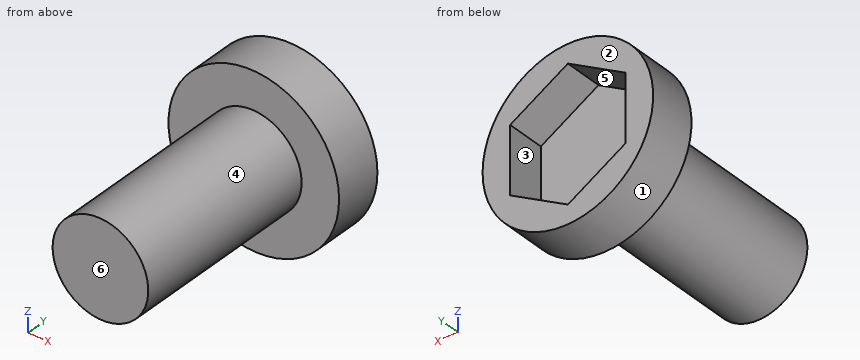
Autodesk Inventor part; units mm, degrees
ref_plane "YZ Plane" through (0, 0, 0) normal (1, 0, 0) x (0, 1, 0)
ref_plane "XZ Plane" through (0, 0, 0) normal (0, 1, 0) x (-1, 0, 0)
ref_plane "XY Plane" through (0, 0, 0) normal (0, 0, 1) x (1, 0, 0)
sketch "Sketch1" plane through (0, 0, 0) normal (0, 1, 0) x (-1, 0, 0)
  circle A0 centre (0, 0) radius 6.35
  dimension "d0" = 12.7
extrude "Extrusion1" add sketch "Sketch1" along normal blind 25.4
thread "Thread1"
sketch "Sketch2" plane through (0, 25.4, 0) normal (0, 1, 0) x (1, 0, 0)
  circle A0 centre (0, 0) radius 11.3208
extrude "Extrusion2" add sketch "Sketch2" along normal blind 6.35
sketch "Sketch3" plane through (0, 31.75, 0) normal (0, 1, 0) x (1, 0, 0)
  line L0 (0, 8.8433) -> (7.6585, 4.4216)
  line L1 (7.6585, 4.4216) -> (7.6585, -4.4216)
  line L2 (7.6585, -4.4216) -> (0, -8.8433)
  line L3 (0, -8.8433) -> (-7.6585, -4.4216)
  line L4 (-7.6585, -4.4216) -> (-7.6585, 4.4216)
  line L5 (-7.6585, 4.4216) -> (0, 8.8433)
  point P0 (0, 0)
  point P1 (0, 0)
extrude "Extrusion3" cut sketch "Sketch3" against normal blind 5.08
properties part number "bolttest"
Design review of the part built by this model. Coordinates are the model's own, in mm. Face numbers are marked on the shaded views. A direction names the side the tool comes from. Round coordinates to 2 decimals unless told otherwise and drop trailing zeros. Loops run counter-clockwise (first coordinate to the right, second up) from the corner with the lowest first, then second, coordinate; pieces in that order, holes last. Notation, with made-up numbers: (84.5, 47) -> (128.5, 47) arc R11 cw to (128.5, 55) -> close; hole circle Ø1 at (28, 72.25). An arc over 180 degrees is marked (long way). Use one line per item in the form item = value. Start each with the question number.
Q1. We need section B-B on z = 0. Give the boundary of the cut face in (x, y).
Q2. We need section C-C on y = 24. Give the boundary of the cut face in (x, z), then the cut area to 3 significant figures.
Q3. Machinability: for the marked faces 4, 5 and 6, which of the approach directions +Z, -Z, +X, -X, +Y, -Y give a long, thin tool a straight path to every point of the face, cutting with its end or side? Answer none if there is none.
Q4. We need section A-A on y = 28. Give the boundary of the cut face in (x, z), then the cut area to 3 significant figures.
Q5. Draft analysis for pull direction X (two halves, no side actions). For the marked faces 1, 2 and 3, state which applies: +X half, -X half, draft (parallel to the pull), parting line (faces both ways), or undercut.
Q6. Wall thickness on line 1 along Y through (x, z) = (2.5, 3.5); line 2 along Y through (x, z) = (-2, 9.5); line 3 along X through (y, z) = (29, -3.5): over which ranges is each line inside the solid? List them lowest first. Write a range as [from, to].
Q7. For pin 1 Ø2.5 at (y, z) = (28.5, -1) entering from +X; pin 2 Ø10 at (y, z) = (17, -2.5) entering from +X; pin 3 Ø3 at (x, y) = (5, 12) entering from -Z; pin 4 Ø3 at (y, z) = (23.5, -7) entering from +X, all flat-tipped, find the tip position at first contact; note any pin that passes through.
Q8. We need section D-D on x = -3.5. Give the boundary of the cut face in (y, z), then the cut area to 3 significant figures.
Calculated:
q1.outline = (-11.32, 25.4) -> (-6.35, 25.4) -> (-6.35, 0) -> (6.35, 0) -> (6.35, 25.4) -> (11.32, 25.4) -> (11.32, 31.75) -> (7.66, 31.75) -> (7.66, 26.67) -> (-7.66, 26.67) -> (-7.66, 31.75) -> (-11.32, 31.75) -> close
q2.outline = circle Ø12.7 at (0, 0)
q2.area = 127 mm²
q3.face_4 = -Y
q3.face_5 = +Y
q3.face_6 = +Z, -Z, +X, -X, -Y
q4.outline = circle Ø22.64 at (0, 0); hole (-7.66, -4.42) -> (0, -8.84) -> (7.66, -4.42) -> (7.66, 4.42) -> (0, 8.84) -> (-7.66, 4.42) -> close
q4.area = 199 mm²
q5.face_1 = parting line
q5.face_2 = draft
q5.face_3 = undercut
q6.line_1 = [0, 26.67]
q6.line_2 = [25.4, 31.75]
q6.line_3 = [-10.77, -7.66], [7.66, 10.77]
q7.pin_1 = 11.32
q7.pin_2 = 6.35
q7.pin_3 = -5.3
q7.pin_4 = 3.17
q8.outline = (0, -5.3) -> (25.4, -5.3) -> (25.4, -10.77) -> (31.75, -10.77) -> (31.75, -6.82) -> (26.67, -6.82) -> (26.67, 6.82) -> (31.75, 6.82) -> (31.75, 10.77) -> (25.4, 10.77) -> (25.4, 5.3) -> (0, 5.3) -> close
q8.area = 337 mm²
